Verification items for the finished model (mm, model axes). A direction names the side the tool comes from. Coordinates: 2 decimals unless noted, no trailing zeros. Loops run counter-clockwise (first coordinate to the right, second up) from the corner with the lowest first, then second, coordinate; pieces in that order, holes last.
Q1. Go/stop test with flat-tipped pins: P1, Ø2, axis at x = -11, z = -53, coming from the +Y side; P2, Ø8, axis at x = -7, z = -20, coming from the -Y side; P3, Ø1, axis at x = -35, z = -7, coming from the -Y side. Record where each tip stops, or that it passes through.
Q2. Sectioned sample at A-A (x = 3). Enter the section's corners in (y, z), then the cut area to 3 significant figures.
Q3. Access from +Z, -Z, +X, -X, +Y, -Y to the whole of each face (thin tool, end or side, straight path). Record for faces 4 (the face through (1, -38, -51.5)), 5 (the face through (0, 2, 3)).
Q4. Sectioned sample at D-D (z = 23.5). Enter the section's corners in (x, y) (3 decimals), then the cut area to 3 significant figures.
Q5. Mould release check, pull along X, two halves, no side actions. Record for faces 1 (the face through (36.425, -3, 1)), 2 (the face through (35.439, -5.203, -50.359)), 3 (the face through (-34.425, -3, 1)): +X half, -X half, draft (parallel to the pull), parting line (faces both ways), or undercut.
Q6. Sectioned sample at C-C (x = -28.5). Enter the section's corners in (y, z), then the cut area to 3 significant figures.
Q7. Sectioned sample at B-B (y = -31.5). Enter the section's corners in (x, z) (3 decimals).
Q8. Material ranges on probe 1 along X at (y, z) = (-2.5, 34.5) (3 decimals); probe 2 along Y at (x, z) = (30, 28); probe 3 along Z at (x, y) = (-8, -45), recorded low to high.
```python
from build123d import *

# Parameters (mm, degrees)
SKETCH1_W            = 68.85
SKETCH1_H            = 107
BOSS_EXTRUDE1_DEPTH  = 2
SKETCH2_W            = 68.85
SKETCH2_H            = 2
BOSS_EXTRUDE2_DEPTH  = 67
CUT_EXTRUDE2_REACH   = 132.855
SKETCH5_W            = 68.85
SKETCH5_H            = 2
BOSS_EXTRUDE3_DEPTH  = 51
SKETCH6_W            = 68.85
SKETCH6_H            = 2
BOSS_EXTRUDE4_DEPTH  = 20.36
BOSS_EXTRUDE5_DEPTH  = 1.5
SKETCH13_W           = 2
SKETCH13_H           = 1.5
BOSS_EXTRUDE8_DEPTH  = 3
CUT_EXTRUDE4_REACH   = 97.75
SKETCH9_R            = 1.75
FILLET1_R            = 1.5
FILLET2_R            = 3
FILLET3_R            = 1.5
FILLET4_R            = 3
CUT_EXTRUDE5_REACH   = 111.975
SKETCH10_R           = 1.75
CHAMFER1_SIZE        = 2
SKETCH11_W           = 2
SKETCH11_H           = 109
BOSS_EXTRUDE6_DEPTH  = 4.5
SKETCH14_W           = 68.85
SKETCH14_H           = 0.5
BOSS_EXTRUDE9_DEPTH  = 2
FILLET5_R            = 2
FILLET6_R            = 4
FILLET8_R            = 4
CUT_EXTRUDE6_DEPTH   = 1
CUT_EXTRUDE7_DEPTH   = 125.986967721
SKETCH17_W           = 68.85
SKETCH17_H           = 2
BOSS_EXTRUDE10_DEPTH = 8.66
SKETCH18_W           = 2
SKETCH18_H           = 68.16
BOSS_EXTRUDE11_DEPTH = 2
SKETCH19_W           = 2
SKETCH19_H           = 68.16
BOSS_EXTRUDE12_DEPTH = 2
FILLET9_R            = 4
FILLET10_R           = 4
FILLET11_R           = 1.5


with BuildPart() as part:
    # Sketch1 → Boss-Extrude1 (new body)
    with BuildSketch(Plane(origin=(0, 0, 0), x_dir=(1, 0, 0), z_dir=(0, 1, 0))):
        Rectangle(SKETCH1_W, SKETCH1_H)
    extrude(amount=BOSS_EXTRUDE1_DEPTH)

    # Sketch2 → Boss-Extrude2 (add)
    with BuildSketch(Plane.XZ):
        with Locations((0, -52.5)):
            Rectangle(SKETCH2_W, SKETCH2_H)
    extrude(amount=BOSS_EXTRUDE2_DEPTH)

    # Sketch4 → Cut-Extrude2 (cut, up to next)
    with BuildSketch(Plane(origin=(0, 0, -53.5), x_dir=(-1, 0, 0), z_dir=(0, 0, -1)), mode=Mode.PRIVATE) as cut_extrude2_sk1:
        Polygon((-6.85, -15.65), (-6.85, -20.95), (-5.325, -20.95), (6.85, -20.95), (6.85, -15.65), (25.15, -15.65), (25.15, -35.75), (-25.15, -35.75), (-25.15, -15.65), align=None)
    cut_extrude2_tool1 = extrude(cut_extrude2_sk1.sketch, amount=-CUT_EXTRUDE2_REACH, mode=Mode.PRIVATE) & part.part
    add(cut_extrude2_tool1.solids().sort_by_distance((0, -26.272573, -53.5))[0], mode=Mode.SUBTRACT)

    # Sketch5 → Boss-Extrude3 (add)
    with BuildSketch(Plane.XY.offset(-51.5)):
        with Locations((0, -66)):
            Rectangle(SKETCH5_W, SKETCH5_H)
    extrude(amount=BOSS_EXTRUDE3_DEPTH)

    # Sketch6 → Boss-Extrude4 (add)
    with BuildSketch(Plane.XZ.offset(67)):
        with Locations((0, -1.5)):
            Rectangle(SKETCH6_W, SKETCH6_H)
    extrude(amount=BOSS_EXTRUDE4_DEPTH)

    # Sketch8 → Boss-Extrude5 (add)
    with BuildSketch(Plane(origin=(0, 2, 0), x_dir=(1, 0, 0), z_dir=(0, 1, 0))):
        Polygon((-36.425, 50.5), (-34.425, 50.5), (-34.425, -53.5), (34.425, -53.5), (34.425, 50.5), (36.425, 50.5), (36.425, -55.5), (-36.425, -55.5), align=None)
    extrude(amount=-BOSS_EXTRUDE5_DEPTH)

    # Sketch13 → Boss-Extrude8 (add)
    with BuildSketch(Plane(origin=(0, 0, -50.5), x_dir=(-1, 0, 0), z_dir=(0, 0, -1))):
        with Locations((35.425, 1.25)):
            Rectangle(SKETCH13_W, SKETCH13_H)
        with Locations((-35.425, 1.25)):
            Rectangle(SKETCH13_W, SKETCH13_H)
    extrude(amount=BOSS_EXTRUDE8_DEPTH)

    # Sketch9 → Cut-Extrude4 (cut, up to next)
    with BuildSketch(Plane.XZ.offset(67), mode=Mode.PRIVATE) as cut_extrude4_sk1:
        with Locations(Location((-25, -23.48, 0), (0, 0, 270))):
            Circle(SKETCH9_R)
    cut_extrude4_tool1 = extrude(cut_extrude4_sk1.sketch, amount=-CUT_EXTRUDE4_REACH, mode=Mode.PRIVATE) & part.part
    # Sketch9 → Cut-Extrude4 (cut, up to next)
    with BuildSketch(Plane.XZ.offset(67), mode=Mode.PRIVATE) as cut_extrude4_sk2:
        with Locations(Location((25, -23.48, 0), (0, 0, 270))):
            Circle(SKETCH9_R)
    cut_extrude4_tool2 = extrude(cut_extrude4_sk2.sketch, amount=-CUT_EXTRUDE4_REACH, mode=Mode.PRIVATE) & part.part
    add(cut_extrude4_tool1.solids().sort_by_distance((-25, -67, -23.48))[0], mode=Mode.SUBTRACT)
    add(cut_extrude4_tool2.solids().sort_by_distance((25, -67, -23.48))[0], mode=Mode.SUBTRACT)

    # Fillet1
    fillet1_edges = [part.edges().sort_by_distance(p)[0] for p in [
        (0, -67, -2.5),
    ]]
    fillet(fillet1_edges, radius=FILLET1_R)

    # Fillet2
    fillet2_edges = [part.edges().sort_by_distance(p)[0] for p in [
        (0, -65, -0.5),
    ]]
    fillet(fillet2_edges, radius=FILLET2_R)

    # Fillet3
    fillet3_edges = [part.edges().sort_by_distance(p)[0] for p in [
        (0, -65, -51.5),
    ]]
    fillet(fillet3_edges, radius=FILLET3_R)

    # Fillet4
    fillet4_edges = [part.edges().sort_by_distance(p)[0] for p in [
        (0, -67, -53.5),
    ]]
    fillet(fillet4_edges, radius=FILLET4_R)

    # Sketch10 → Cut-Extrude5 (cut, up to next)
    with BuildSketch(Plane.XY.offset(-0.5), mode=Mode.PRIVATE) as cut_extrude5_sk1:
        with Locations((-24.425, -79.36)):
            Circle(SKETCH10_R)
    cut_extrude5_tool1 = extrude(cut_extrude5_sk1.sketch, amount=-CUT_EXTRUDE5_REACH, mode=Mode.PRIVATE) & part.part
    # Sketch10 → Cut-Extrude5 (cut, up to next)
    with BuildSketch(Plane.XY.offset(-0.5), mode=Mode.PRIVATE) as cut_extrude5_sk2:
        with Locations((24.425, -79.36)):
            Circle(SKETCH10_R)
    cut_extrude5_tool2 = extrude(cut_extrude5_sk2.sketch, amount=-CUT_EXTRUDE5_REACH, mode=Mode.PRIVATE) & part.part
    add(cut_extrude5_tool1.solids().sort_by_distance((-24.425, -79.36, -0.5))[0], mode=Mode.SUBTRACT)
    add(cut_extrude5_tool2.solids().sort_by_distance((24.425, -79.36, -0.5))[0], mode=Mode.SUBTRACT)

    # Chamfer1
    chamfer1_edges = [part.edges().sort_by_distance(p)[0] for p in [
        (-34.425, -87.36, -1.5),
        (34.425, -87.36, -1.5),
    ]]
    chamfer(chamfer1_edges, length=CHAMFER1_SIZE)

    # Sketch11 → Boss-Extrude6 (add)
    with BuildSketch(Plane.XZ.offset(-0.5)):
        with Locations((35.425, 1)):
            Rectangle(SKETCH11_W, SKETCH11_H)
        with Locations((-35.425, 1)):
            Rectangle(SKETCH11_W, SKETCH11_H)
    extrude(amount=BOSS_EXTRUDE6_DEPTH)

    # Sketch14 → Boss-Extrude9 (add)
    with BuildSketch(Plane.XY.offset(53.5)):
        with Locations((0, 0.25)):
            Rectangle(SKETCH14_W, SKETCH14_H)
    extrude(amount=BOSS_EXTRUDE9_DEPTH)

    # Fillet5
    fillet5_edges = [part.edges().sort_by_distance(p)[0] for p in [
        (0, 0, -51.5),
        (34.425, 0, 2),
        (-34.425, 0, 2),
    ]]
    fillet(fillet5_edges, radius=FILLET5_R)

    # Fillet6
    fillet6_edges = [part.edges().sort_by_distance(p)[0] for p in [
        (0, 2, -53.5),
    ]]
    fillet(fillet6_edges, radius=FILLET6_R)

    # Fillet8
    # the kernel refuses this fillet: 4 mm, written as the material it takes off along each edge
    with BuildSketch(Plane(origin=(-36.425, 2, 65.5), x_dir=(1, 0, 0), z_dir=(0, 0, -1))) as fillet8_piece_1:
        with BuildLine():
            CenterArc((FILLET8_R, FILLET8_R), FILLET8_R, 180, 90)
            Line((0, FILLET8_R), (0, 0))
            Line((0, 0), (FILLET8_R, 0))
        make_face()
    extrude(amount=125, mode=Mode.SUBTRACT)
    with BuildSketch(Plane(origin=(36.425, 2, -59.5), x_dir=(0, -1, 0), z_dir=(0, 0, 1))) as fillet8_piece_2:
        with BuildLine():
            CenterArc((FILLET8_R, -FILLET8_R), FILLET8_R, 90, 90)
            Line((0, -FILLET8_R), (0, 0))
            Line((0, 0), (FILLET8_R, 0))
        make_face()
    extrude(amount=125, mode=Mode.SUBTRACT)

    # Sketch15 → Cut-Extrude6 (cut)
    with BuildSketch(Plane.XY.offset(55.5)):
        with BuildLine():
            Line((-36.425, -2), (-36.425, -4))
            Line((-36.425, -4), (-34.425, -4))
            Line((-34.425, -4), (-34.425, -2))
            ThreePointArc((-34.425, -2), (-33.839213562, -0.585786438), (-32.425, 0))
            Line((-32.425, 0), (32.425, 0))
            ThreePointArc((32.425, 0), (33.839213562, -0.585786438), (34.425, -2))
            Line((34.425, -2), (34.425, -4))
            Line((34.425, -4), (36.425, -4))
            Line((36.425, -4), (36.425, -2))
            ThreePointArc((36.425, -2), (35.253427125, 0.828427125), (32.425, 2))
            Line((32.425, 2), (-32.425, 2))
            ThreePointArc((-32.425, 2), (-35.253427125, 0.828427125), (-36.425, -2))
        make_face()
    extrude(amount=-CUT_EXTRUDE6_DEPTH, mode=Mode.SUBTRACT)

    # Sketch16 → Cut-Extrude7 (cut, through all)
    with BuildSketch(Plane(origin=(34.425, 0, 0), x_dir=(0, 0, -1), z_dir=(1, 0, 0))):
        with BuildLine():
            Line((2.5, -87.36), (0.5, -87.36))
            Line((0.5, -87.36), (0.5, -68))
            ThreePointArc((0.5, -68), (1.378679656, -65.878679656), (3.5, -65))
            Line((3.5, -65), (50, -65))
            ThreePointArc((50, -65), (51.060660172, -64.560660172), (51.5, -63.5))
            Line((51.5, -63.5), (53.5, -63.5))
            Line((53.5, -63.5), (53.5, -64))
            ThreePointArc((53.5, -64), (52.621320344, -66.121320344), (50.5, -67))
            Line((50.5, -67), (4, -67))
            ThreePointArc((4, -67), (2.939339828, -67.439339828), (2.5, -68.5))
            Line((2.5, -68.5), (2.5, -87.36))
        make_face()
    extrude(amount=-CUT_EXTRUDE7_DEPTH, mode=Mode.SUBTRACT)

    # Sketch17 → Boss-Extrude10 (add)
    with BuildSketch(Plane.XZ.offset(63.5)):
        with Locations((0, -52.5)):
            Rectangle(SKETCH17_W, SKETCH17_H)
    extrude(amount=BOSS_EXTRUDE10_DEPTH)

    # Sketch18 → Boss-Extrude11 (add)
    with BuildSketch(Plane(origin=(34.425, 0, 0), x_dir=(0, 0, -1), z_dir=(1, 0, 0))):
        with Locations((52.5, -38.08)):
            Rectangle(SKETCH18_W, SKETCH18_H)
    extrude(amount=BOSS_EXTRUDE11_DEPTH)

    # Sketch19 → Boss-Extrude12 (add)
    with BuildSketch(Plane.ZY.offset(34.425)):
        with Locations((-52.5, -38.08)):
            Rectangle(SKETCH19_W, SKETCH19_H)
    extrude(amount=BOSS_EXTRUDE12_DEPTH)

    # Fillet9
    fillet9_edges = [part.edges().sort_by_distance(p)[0] for p in [
        (36.425, -72.16, -52.5),
        (-36.425, -72.16, -52.5),
    ]]
    fillet(fillet9_edges, radius=FILLET9_R)

    # Fillet10
    fillet10_edges = [part.edges().sort_by_distance(p)[0] for p in [
        (35.425, -4, -51.5),
        (-35.425, -4, -51.5),
    ]]
    fillet(fillet10_edges, radius=FILLET10_R)

    # Fillet11
    fillet11_edges = [part.edges().sort_by_distance(p)[0] for p in [
        (35.425, -4, 54.5),
        (-35.425, -4, 54.5),
    ]]
    fillet(fillet11_edges, radius=FILLET11_R)


solid = part.part
```
Geometry check:
1. P1: stops at y = 1.12
1. P2: stops at y = 0
1. P3: stops at y = -4
2. outline: (-72.16, -53.5) - (-35.75, -53.5) - (-35.75, -51.5) - (-72.16, -51.5) - close; (-20.95, -53.5) - (-2, -53.5) arc R4 ccw to (2, -49.5) - (2, 54.5) - (0, 54.5) - (0, -49.5) arc R2 cw to (-2, -51.5) - (-20.95, -51.5) - close
2. area: 328 mm2
3. face 4: +Z, -Y
3. face 5: +Z, -Z, +X, -X, +Y
4. outline: (-36.425, -4) - (-34.425, -4) - (-34.425, -2) arc R2 cw to (-32.425, 0) - (32.425, 0) arc R2 cw to (34.425, -2) - (34.425, -4) - (36.425, -4) - (36.425, -2) arc R4 ccw to (32.425, 2) - (-32.425, 2) arc R4 ccw to (-36.425, -2) - close
4. area: 157 mm2
5. face 1: +X half
5. face 2: draft
5. face 3: undercut
6. outline: (-72.16, -53.5) - (-2, -53.5) arc R4 ccw to (2, -49.5) - (2, 54.5) - (0, 54.5) - (0, -49.5) arc R2 cw to (-2, -51.5) - (-72.16, -51.5) - close
6. area: 358 mm2
7. outline: (-36.425, -53.5) - (-25.15, -53.5) - (-25.15, -51.5) - (-36.425, -51.5) - close; (25.15, -53.5) - (36.425, -53.5) - (36.425, -51.5) - (25.15, -51.5) - close
8. probe 1: x = -36.425 to -34.425, 34.425 to 36.425
8. probe 2: y = 0 to 2
8. probe 3: z = -53.5 to -51.5
